```python
from build123d import *

# Parameters (mm, degrees)
F1_DEPTH = 5
F2_R     = 2
F3_R     = 2
F4_DEPTH = 5
F5_W     = 20
F5_H     = 4
F6_DEPTH = 20


with BuildPart() as f1:
    # F0 (on Top) → F1 (new body)
    with BuildSketch(Plane.XY):
        with BuildLine():
            ThreePointArc((-40, 70.154987), (30.639398, 73.914586), (0, 10.154987))
            Line((0, 10.154987), (-100, 10.154987))
            Line((-100, 10.154987), (-100, 0))
            Line((-100, 0), (-3.517851, 0))
            ThreePointArc((-3.517851, 0), (43.563989, 70.884062), (-40, 86.956077))
            Line((-40, 86.956077), (-40, 70.154987))
        make_face()
    extrude(amount=F1_DEPTH)

    # F2
    f2_edges = [f1.edges().sort_by_distance(p)[0] for p in [
        (-40, 70.154987, 2.5),
        (-40, 86.956077, 2.5),
    ]]
    fillet(f2_edges, radius=F2_R)

    # F3 (on face) → F4 (cut)
    with BuildSketch(Plane.XY.offset(5)):
        with Locations((-36.878993, 80.881587)):
            Circle(F3_R)
        with Locations((-20.412356, 91.712579)):
            Circle(F3_R)
        with Locations((-9.581419, 94.495535)):
            Circle(F3_R)
        with Locations((-29.287707, 87.124474)):
            Circle(F3_R)
        with Locations((-11.243654, 5.575917)):
            Circle(F3_R)
        with Locations((14.160543, 10.102125)):
            Circle(F3_R)
        with Locations((26.199445, 17.886208)):
            Circle(F3_R)
        with Locations((1.5747, 6.171187)):
            Circle(F3_R)
    extrude(amount=-F4_DEPTH, mode=Mode.SUBTRACT)

    # F5 (on face) → F6 (join)
    with BuildSketch(Plane.XY.offset(5)):
        with Locations((-37.5, 2)):
            Rectangle(F5_W, F5_H)
        with Locations((-87.5, 2)):
            Rectangle(F5_W, F5_H)
    extrude(amount=-F6_DEPTH)


solid = f1.part
```
Work out the finished part from the listing and answer in its coordinate system (mm). A direction names the side the tool comes from. Give positions to 0.01 mm unless a question says otherwise; leave off trailing zeros. Write each loop counter-clockwise with the first axis right and the second up, starting at its lowest first coordinate (ties: lowest second). Pieces come first, ordered by that corner, then holes. Notation, with made-up numbers: (-21, 72.25) - (1, 72.25) arc R18 cw to (1, 106.25) - close; hole circle Ø1 at (66.5, 73.5). An arc over 180 degrees is marked (long way). Use one line per item in the form item = value.
1. Consider L1, parallel to Y at x = -81, z = -10; L2, parallel to Z at x = 35, y = 22; L3, parallel to X at y = 96, z = 3.25. Determine where each line is inside the solid, lowest interval first.
Filled in:
L1 = 0 to 4
L2 = 0 to 5
L3 = -28 to -10.9, -8.26 to 20.87
2. A cutting plane is placed at A-A (z = -8). Write down the section's boundary in (x, y).
Filled in:
outline = (-97.5, 0) - (-77.5, 0) - (-77.5, 4) - (-97.5, 4) - close; (-47.5, 0) - (-27.5, 0) - (-27.5, 4) - (-47.5, 4) - close
3. A cutting plane is placed at D-D (x = 26). Write down the section's boundary in (y, z).
Filled in:
outline = (9.42, 0) - (15.9, 0) - (15.9, 5) - (9.42, 5) - close; (19.88, 0) - (22.55, 0) - (22.55, 5) - (19.88, 5) - close; (79.67, 0) - (92.8, 0) - (92.8, 5) - (79.67, 5) - close
4. For faces 1 (the face through (-47.5, 2, -7)), 2 (the face through (-38, 4, -7)), 3 (the face through (-49, 10.155, 2)), 4 (the face through (-38, 2, -15)), determine the directions among +Z, -Z, +X, -X, +Y, -Y from which every point of the face is accessible in a straight line to the end or side of a thin tool.
Filled in:
face_1 = -Z, +Y, -Y
face_2 = -Z, +X, -X, +Y
face_3 = +Z, -Z, -X
face_4 = -Z, +X, -X, +Y, -Y
5. Each of these flat-tipped pins is pushed along its axis until it touches: pin 1 Ø4.5 at (y, z) = (3, -8) entering from +X; pin 2 Ø4 at (x, z) = (-47, -7.5) entering from +Y; pin 3 Ø6 at (y, z) = (46.5, 2.5) entering from +X. Where does it stop, or does it pass through?
Filled in:
pin_1 = -27.5
pin_2 = 4
pin_3 = 47.52
6. A cutting plane is placed at B-B (x = -24.5). Write down the section's boundary in (y, z), and give its area (3 significant figures).
Filled in:
outline = (0, 0) - (10.15, 0) - (10.15, 5) - (0, 5) - close; (86.49, 0) - (97.74, 0) - (97.74, 5) - (86.49, 5) - close
area = 107 mm^2
7. A cutting plane is placed at C-C (z = 3.5). State how many separate pieces and enclosed holes the cut face has, and give its area (3 significant figures).
Filled in:
separate_pieces = 1
enclosed_holes = 8
area = 2,740 mm^2
8. Determine the mould class of faces 5 (the face through (-27.5, 2, -7)), 6 (the face through (-88, 4, -7)), 7 (the face through (-40, 82, 2)), 8 (the face through (24.61, 16.67, 2.54)) for opening direction X: released by +X, released by -X, zero draft, split by the parting line, or undercut.
Filled in:
face_5 = released by +X
face_6 = zero draft
face_7 = released by -X
face_8 = undercut
